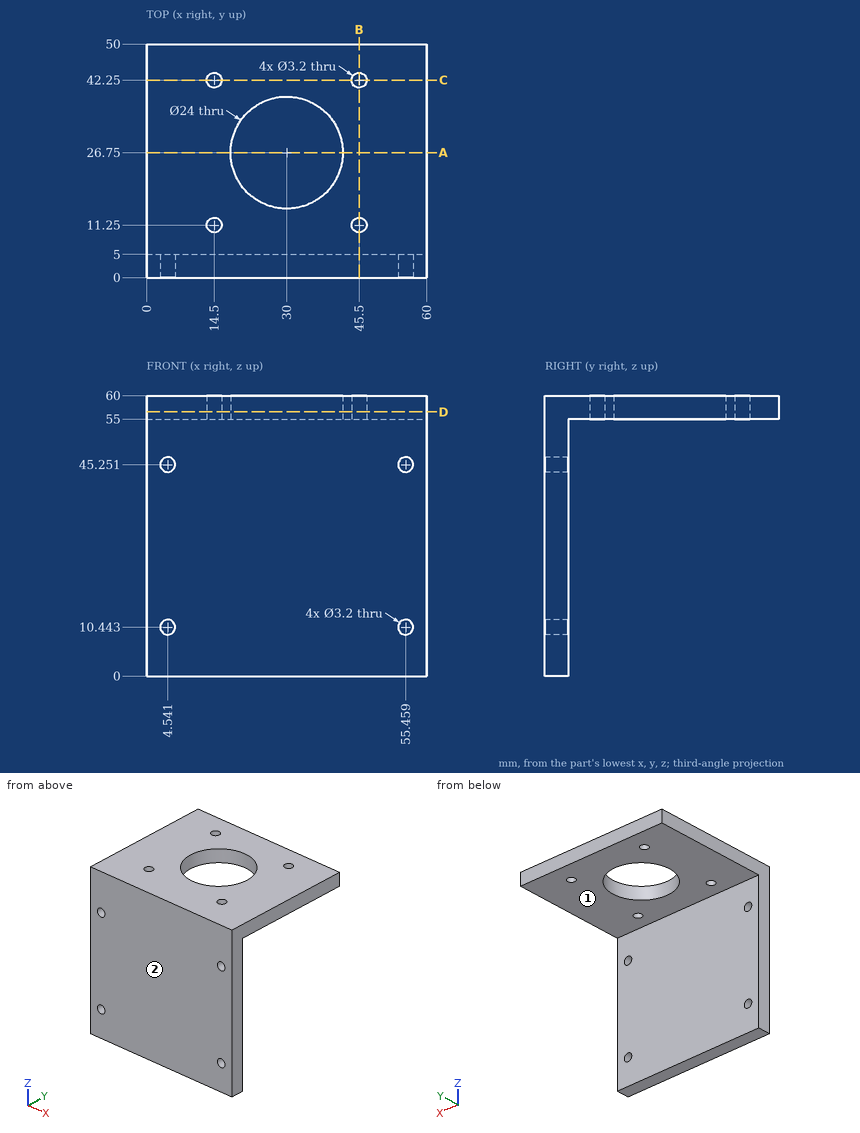
Geometry check sheet. Reference: drawing and pictorial views, mm from the part's lowest x, y, z. A direction names the side the tool comes from. Coordinates: 2 decimals unless noted, no trailing zeros. Order: outer loops, then holes, each group sorted by start corner. A loop starts at its lowest first (then second) coordinate and runs counter-clockwise, first axis right, second up. Notation, with made-up numbers: (25, 46.25) -> (33, 46.25) arc R30 cw to (33, 85.25) -> close; hole circle Ø6 at (17.5, -25). An arc over 180 degrees is marked (long way). Write item = value, one per line. Start each with the question number.
1) Cross-section at D-D (z = 56.5). Enter the section's corners in (x, y), then the cut area to 3 significant figures.
2) Cross-section at C-C (y = 42.25). Enter the section's corners in (x, z).
3) Material ranges on L1, parallel to Y at x = 14.5, z = 57.1; L2, parallel to Y at x = 30, z = 58.8; L3, parallel to Z at x = 14, y = 16.5, recorded low to high.
4) Cross-section at B-B (x = 45.5). Enter the section's corners in (y, z), then the cut area to 3 significant figures.
5) Access from +Z, -Z, +X, -X, +Y, -Y to the whole of each face (thin tool, end or side, straight path). Record for the marked faces 1 and 2.
6) Cross-section at A-A (y = 26.75). Enter the section's corners in (x, z).
7) Go/stop test with flat-tipped pins: P1, Ø4, axis at x = 14.5, y = 42.25, coming from the -Z side; P2, Ø5, axis at x = 39.5, z = 25, coming from the +Y side. Record where each tip stops, or that it passes through.
Ans:
q1.outline = (0, 0) -> (60, 0) -> (60, 50) -> (0, 50) -> close; hole circle Ø3.2 at (14.5, 11.25); hole circle Ø3.2 at (14.5, 42.25); hole circle Ø24 at (30, 26.75); hole circle Ø3.2 at (45.5, 11.25); hole circle Ø3.2 at (45.5, 42.25)
q1.area = 2,520 mm²
q2.outline = (0, 55) -> (12.9, 55) -> (12.9, 60) -> (0, 60) -> close; (16.1, 55) -> (43.9, 55) -> (43.9, 60) -> (16.1, 60) -> close; (47.1, 55) -> (60, 55) -> (60, 60) -> (47.1, 60) -> close
q3.L1 = 0 to 9.65, 12.85 to 40.65, 43.85 to 50
q3.L2 = 0 to 14.75, 38.75 to 50
q3.L3 = 55 to 60
q4.outline = (0, 0) -> (5, 0) -> (5, 55) -> (9.65, 55) -> (9.65, 60) -> (0, 60) -> close; (12.85, 55) -> (40.65, 55) -> (40.65, 60) -> (12.85, 60) -> close; (43.85, 55) -> (50, 55) -> (50, 60) -> (43.85, 60) -> close
q4.area = 493 mm²
q5.face_1 = -Z, +X, -X, +Y
q5.face_2 = +Z, -Z, +X, -X, -Y
q6.outline = (0, 55) -> (18, 55) -> (18, 60) -> (0, 60) -> close; (42, 55) -> (60, 55) -> (60, 60) -> (42, 60) -> close
q7.P1 = 55
q7.P2 = 5
